from build123d import *

# Parameters (mm, degrees)
ESQUISSE1_W             = 30
ESQUISSE1_H             = 67
ESQUISSE1_R             = 4
BOSS_EXTRU_1_DEPTH      = 5
ESQUISSE2_W             = 30
ESQUISSE2_H             = 12.5
ENL_V_MAT_EXTRU_1_DEPTH = 5
ESQUISSE3_W             = 5
ESQUISSE3_H             = 5
ENL_V_MAT_EXTRU_2_DEPTH = 38.043892884
BOSS_EXTRU_2_DEPTH      = 5
ENL_V_MAT_EXTRU_3_DEPTH = 40.33509883
ESQUISSE8_W             = 41.113396405
ESQUISSE8_H             = 1
ENL_V_MAT_EXTRU_4_DEPTH = 40.33509883
CONG_1_R                = 10
CONG_2_R                = 10


with BuildPart() as part:
    # Esquisse1 → Boss.-Extru.1 (new body)
    with BuildSketch(Plane.XY):
        Rectangle(ESQUISSE1_W, ESQUISSE1_H)
        with Locations((0, 12.5)):
            Circle(ESQUISSE1_R, mode=Mode.SUBTRACT)
    extrude(amount=BOSS_EXTRU_1_DEPTH)

    # Esquisse2 → Enlèv. mat.-Extru.1 (cut)
    with BuildSketch(Plane.XY.offset(5)):
        with Locations((0, 27.25)):
            Rectangle(ESQUISSE2_W, ESQUISSE2_H)
    extrude(amount=-ENL_V_MAT_EXTRU_1_DEPTH, mode=Mode.SUBTRACT)

    # Esquisse3 → Enlèv. mat.-Extru.2 (cut, through all)
    with BuildSketch(Plane.XY.offset(5)):
        with Locations((-10.5, -31)):
            Rectangle(ESQUISSE3_W, ESQUISSE3_H)
        with Locations((10.5, -31)):
            Rectangle(ESQUISSE3_W, ESQUISSE3_H)
    extrude(amount=-ENL_V_MAT_EXTRU_2_DEPTH, mode=Mode.SUBTRACT)

    # Esquisse5 → Boss.-Extru.2 (add)
    with BuildSketch(Plane.XY.offset(5)):
        Polygon((-15, -19.875), (-20, -33.5), (-15, -33.5), align=None)
        Polygon((15, -19.875), (20, -33.5), (15, -33.5), align=None)
    extrude(amount=-BOSS_EXTRU_2_DEPTH)

    # Esquisse6 → Enlèv. mat.-Extru.3 (cut, through all)
    with BuildSketch(Plane.XY.offset(5)):
        Polygon((-15, 10.78125), (-5, 21), (-15, 21), align=None)
        Polygon((15, 10.78125), (5, 21), (15, 21), align=None)
    extrude(amount=-ENL_V_MAT_EXTRU_3_DEPTH, mode=Mode.SUBTRACT)

    # Esquisse8 → Enlèv. mat.-Extru.4 (cut, through all)
    with BuildSketch(Plane.XY.offset(5)):
        with Locations((0.556698202, -33)):
            Rectangle(ESQUISSE8_W, ESQUISSE8_H)
    extrude(amount=-ENL_V_MAT_EXTRU_4_DEPTH, mode=Mode.SUBTRACT)

    # Congé1
    cong_1_edges = [part.edges().sort_by_distance(p)[0] for p in [
        (-15, 10.78125, 2.5),
        (-5, 21, 2.5),
        (15, 10.78125, 2.5),
        (5, 21, 2.5),
    ]]
    fillet(cong_1_edges, radius=CONG_1_R)

    # Congé2
    cong_2_edges = [part.edges().sort_by_distance(p)[0] for p in [
        (-15, -19.875, 2.5),
        (15, -19.875, 2.5),
    ]]
    fillet(cong_2_edges, radius=CONG_2_R)


solid = part.part
Input: part model. Units: mm. Frame: model coordinates. A direction names the side the tool comes from. Round coordinates to 2 decimals unless told otherwise and drop trailing zeros. Order: outer loops, then holes, each group sorted by start corner. A loop starts at its lowest first (then second) coordinate and runs counter-clockwise, first axis right, second up. Notation, with made-up numbers: (88, -12) - (124, -12) arc R21 ccw to (124, 2) - close; hole circle Ø11 at (28.5, 54.5). An arc over 180 degrees is marked (long way). Answer as a JSON object with one key per item and string values. Group by question number.
(1) Material intervals for probe 1 along Y at (x, z) = (0, 3.75); probe 2 along X at (y, z) = (18, 2.85); probe 3 along X at (y, z) = (-10, 2.5), sorted ascending. Write a range as from..to.
(2) Draft query along Y for faces 1 (the face through (-14.28, 10.43, 2.46)), 2 (the face through (10, -28.5, 3)), 3 (the face through (-0.521, 16.466, 2.465)), 4 (the face through (0, -5, 0)). Return one class per face: released by +Y, released by -Y, zero draft, split by the parting line, or undercut.
(3) Reachability of faces 5 (the face through (-11, -28.5, 3)), 6 (the face through (0, -5, 5)), 7 (the face through (-15, -6, 2)), 8 (the face through (15, -6, 2)) from +Z, -Z, +X, -X, +Y, -Y: full face, straight path, thin tool, end or side. Return the list, or none.
(4) Cut plane A-A (x = 0). Return loops of the section in (y, z), then the cut area to 4 significant figures.
(5) Cut plane B-B (z = 0.95). Return loops of the section in (x, y), then the cut area to 3 significant figures.
(6) Pin query (flat end, axial travel): P1, Ø1.5, axis at x = 12, z = 0.5, coming from the -Y side; P2, Ø1.2, axis at y = -30, z = 3, coming from the +X side; P3, Ø3, axis at y = -30, z = 2, coming from the -X side. Return the tip coordinate at first contact, or that it passes through.
(7) Cut plane C-C (y = 15.5). Return loops of the section in (x, z).
(8) Cut plane D-D (y = 3). Return loops of the section in (x, z).
Here are the results:
{
 "1": {"probe 1": "y = -32.5..8.5, 16.5..21", "probe 2": "x = -7.94..7.94", "probe 3": "x = -15..15"},
 "2": {"face 1": "released by +Y", "face 2": "released by -Y", "face 3": "undercut", "face 4": "zero draft"},
 "3": {"face 5": "+Z, -Z, -Y", "face 6": "+Z, +X, -X, +Y, -Y", "face 7": "+Z, -Z, -X, +Y", "face 8": "+Z, -Z, +X, +Y"},
 "4": {"outline": "(-32.5, 0) - (8.5, 0) - (8.5, 5) - (-32.5, 5) - close; (16.5, 0) - (21, 0) - (21, 5) - (16.5, 5) - close", "area": "227.5 mm^2"},
 "5": {"outline": "(-19.63, -32.5) - (-13, -32.5) - (-13, -28.5) - (-8, -28.5) - (-8, -32.5) - (8, -32.5) - (8, -28.5) - (13, -28.5) - (13, -32.5) - (19.63, -32.5) - (15.61, -21.54) arc R10 cw to (15, -18.1) - (15, 6.7) arc R10 ccw to (12.15, 13.7) - (7.94, 17.99) arc R10 ccw to (0.79, 21) - (-0.79, 21) arc R10 ccw to (-7.94, 17.99) - (-12.15, 13.7) arc R10 ccw to (-15, 6.7) - (-15, -18.1) arc R10 cw to (-15.61, -21.54) - close; hole circle Ø8 at (0, 12.5)", "area": "1,460 mm^2"},
 "6": {"P1": "stops at y = -28.5", "P2": "stops at x = 18.94", "P3": "stops at x = -19.27"},
 "7": {"outline": "(-10.38, 0) - (-2.65, 0) - (-2.65, 5) - (-10.38, 5) - close; (2.65, 0) - (10.38, 0) - (10.38, 5) - (2.65, 5) - close"},
 "8": {"outline": "(-15, 0) - (15, 0) - (15, 5) - (-15, 5) - close"}
}
